CAD build for the part. Positions are in the model's coordinates, mm. Face numbers are marked on the shaded views. A direction names the side the tool comes from. Round coordinates to 2 decimals unless told otherwise and drop trailing zeros. Loops run counter-clockwise (first coordinate to the right, second up) from the corner with the lowest first, then second, coordinate; pieces in that order, holes last.
from build123d import *

# Parameters (mm, degrees)
SKETCH_1_W           = 50
SKETCH_1_H           = 50
EXTRUDE_1_DEPTH      = 220
EXTRUDE_2_DEPTH      = 50
SKETCH_4_W           = 37
SKETCH_4_H           = 37
CUT_EXTRUDE_2_DEPTH  = 12
CUT_EXTRUDE_3_REACH  = 235.922
SKETCH_5_R           = 8.5
SKETCH_8_R           = 0.75
CUT_EXTRUDE_4_DEPTH  = 6.5
CUT_EXTRUDE_START    = -6.5
SKETCH_7_R           = 0.75
CUT_EXTRUDE_5_DEPTH  = 6.5
CUT_EXTRUDE_6_DEPTH  = 5.5
CUT_EXTRUDE_7_DEPTH  = 5.5
CUT_EXTRUDE_8_DEPTH  = 50
FILLET_1_R           = 5
FILLET_2_R           = 5
FILLET_3_R           = 10
FILLET_4_R           = 10
SKETCH_13_W          = 47
SKETCH_13_H          = 47
CUT_EXTRUDE_9_DEPTH  = 50
SKETCH_2_W           = 43
SKETCH_2_H           = 43
CUT_EXTRUDE_10_DEPTH = 150
FILLET_5_R           = 5


with BuildPart() as part:
    # 草图1 → 凸台-拉伸1 (new body)
    with BuildSketch(Plane.XY):
        Rectangle(SKETCH_1_W, SKETCH_1_H)
    extrude(amount=EXTRUDE_1_DEPTH)

    # 草图3 → 凸台-拉伸2 (add)
    with BuildSketch(Plane(origin=(0, 25, 0), x_dir=(1, 0, 0), z_dir=(0, 1, 0))):
        Polygon((25, 0), (-25, 0), (26.961524227, 30), (76.961524227, 30), align=None)
    extrude(amount=-EXTRUDE_2_DEPTH)

    # 草图4 → 切除-拉伸2 (cut)
    with BuildSketch(Plane(origin=(6.25, 0, 10.825317547), x_dir=(0.8660254037844415, 0, -0.4999999999999951), z_dir=(0.4999999999999951, 0, 0.8660254037844415))):
        with Locations((41.650635095, 0)):
            Rectangle(SKETCH_4_W, SKETCH_4_H)
    extrude(amount=-CUT_EXTRUDE_2_DEPTH, mode=Mode.SUBTRACT)

    # 切除-拉伸3: up to this face of the body (flat: up to its plane)
    cut_extrude_3_end = Plane(part.part.faces().sort_by_distance((0.980762114, 0, -15))[0])
    # 草图5 → 切除-拉伸3 (cut, up to the picked face)
    with BuildSketch(Plane(origin=(0.25, 0, 0.433012702), x_dir=(0.8660254037844415, 0, -0.4999999999999951), z_dir=(0.4999999999999951, 0, 0.8660254037844415)), mode=Mode.PRIVATE) as cut_extrude_3_sk1:
        with Locations((45.150635095, 0)):
            Circle(SKETCH_5_R)
    cut_extrude_3_tool1 = split(extrude(cut_extrude_3_sk1.sketch, amount=-CUT_EXTRUDE_3_REACH, mode=Mode.PRIVATE), bisect_by=cut_extrude_3_end, keep=Keep.BOTH, mode=Mode.PRIVATE)
    add(cut_extrude_3_tool1.solids().sort_by(Axis((39.351597, 0, -22.142305), (-0.4999999999999951, 0, -0.8660254037844415)))[0], mode=Mode.SUBTRACT)

    # 草图8 → 切除-拉伸4 (cut)
    with BuildSketch(Plane.XZ.offset(-18.5)):
        with Locations((39.170508076, -15.455960044)):
            Circle(SKETCH_8_R)
    extrude(amount=-CUT_EXTRUDE_4_DEPTH, mode=Mode.SUBTRACT)

    # 草图7 → 切除-拉伸5 (cut)
    with BuildSketch(Plane(origin=(0, -18.5, 0), x_dir=(1, 0, 0), z_dir=(0, 1, 0)).offset(CUT_EXTRUDE_START)):
        with Locations((39.170508076, 15.455960044)):
            Circle(SKETCH_7_R)
    extrude(amount=CUT_EXTRUDE_5_DEPTH, mode=Mode.SUBTRACT)

    # 草图10 → 切除-拉伸6 (cut)
    with BuildSketch(Plane.XZ.offset(25)):
        Polygon((58.341978046, -19.25), (26.299038106, -0.75), (20.299038106, -11.142304845), (52.341978046, -29.642304845), align=None)
    extrude(amount=-CUT_EXTRUDE_6_DEPTH, mode=Mode.SUBTRACT)

    # 草图11 → 切除-拉伸7 (cut)
    with BuildSketch(Plane(origin=(0, 25, 0), x_dir=(1, 0, 0), z_dir=(0, 1, 0))):
        Polygon((26.299038106, 0.75), (58.341978046, 19.25), (52.341978046, 29.642304845), (20.299038106, 11.142304845), align=None)
    extrude(amount=-CUT_EXTRUDE_7_DEPTH, mode=Mode.SUBTRACT)

    # 草图12 → 切除-拉伸8 (cut)
    with BuildSketch(Plane.XZ.offset(25)):
        Polygon((64.404155872, -22.75), (60.218366421, -30), (76.961524227, -30), align=None)
    extrude(amount=-CUT_EXTRUDE_8_DEPTH, mode=Mode.SUBTRACT)

    # 圆角1
    fillet_1_edges = [part.edges().sort_by_distance(p)[0] for p in [
        (60.218366421, 0, -30),
    ]]
    fillet(fillet_1_edges, radius=FILLET_1_R)

    # 圆角2
    fillet_2_edges = [part.edges().sort_by_distance(p)[0] for p in [
        (26.961524227, -15.049152987, -30),
    ]]
    fillet(fillet_2_edges, radius=FILLET_2_R)

    # 圆角3
    fillet_3_edges = [part.edges().sort_by_distance(p)[0] for p in [
        (-25, 0, 0),
    ]]
    fillet(fillet_3_edges, radius=FILLET_3_R)

    # 圆角4
    # the kernel refuses this fillet: 10 mm, written as the material it adds along each edge
    with BuildSketch(Plane(origin=(25, 25, 0), x_dir=(0, 0, 1), z_dir=(0, -1, 0))) as fillet_4_piece_1_section:
        with BuildLine():
            CenterArc((FILLET_4_R * 0.57735026919, -FILLET_4_R), FILLET_4_R, 90, 60)
            Line((-FILLET_4_R * 0.288675134595, -FILLET_4_R * 0.5), (0, 0))
            Line((0, 0), (FILLET_4_R * 0.57735026919, 0))
        make_face()
    fillet_4_piece_1 = extrude(amount=50, mode=Mode.PRIVATE)
    fillet_4_piece_1 = split(fillet_4_piece_1, bisect_by=Plane(origin=(26.950281618, 22.25, 0.377986851), z_dir=(-0.8660254037844415, 0, 0.49999999999999517)), keep=Keep.TOP, mode=Mode.PRIVATE)
    add(fillet_4_piece_1)
    with BuildSketch(Plane(origin=(25, 39.43375673, 0), x_dir=(0, 0, 1), z_dir=(0, -1, 0))) as fillet_4_piece_2_section:
        with BuildLine():
            CenterArc((FILLET_4_R * 0.57735026919, -FILLET_4_R), FILLET_4_R, 90, 60)
            Line((-FILLET_4_R * 0.288675134595, -FILLET_4_R * 0.5), (0, 0))
            Line((0, 0), (FILLET_4_R * 0.57735026919, 0))
        make_face()
    fillet_4_piece_2 = extrude(amount=78.867513459, mode=Mode.PRIVATE)
    fillet_4_piece_2 = split(fillet_4_piece_2, bisect_by=Plane(origin=(27.357776316, 19.5, -1.0319296), z_dir=(0, -1, 0)), keep=Keep.TOP, mode=Mode.PRIVATE)
    fillet_4_piece_2 = split(fillet_4_piece_2, bisect_by=Plane(origin=(27.357776316, 18.5, -1.0319296), z_dir=(0, 1, 0)), keep=Keep.TOP, mode=Mode.PRIVATE)
    add(fillet_4_piece_2)
    with BuildSketch(Plane(origin=(25, 39.43375673, 0), x_dir=(0, 0, 1), z_dir=(0, -1, 0))) as fillet_4_piece_3_section:
        with BuildLine():
            CenterArc((FILLET_4_R * 0.57735026919, -FILLET_4_R), FILLET_4_R, 90, 60)
            Line((-FILLET_4_R * 0.288675134595, -FILLET_4_R * 0.5), (0, 0))
            Line((0, 0), (FILLET_4_R * 0.57735026919, 0))
        make_face()
    fillet_4_piece_3 = extrude(amount=78.867513459, mode=Mode.PRIVATE)
    fillet_4_piece_3 = split(fillet_4_piece_3, bisect_by=Plane(origin=(27.357776316, -19.5, -1.0319296), z_dir=(0, 1, 0)), keep=Keep.TOP, mode=Mode.PRIVATE)
    fillet_4_piece_3 = split(fillet_4_piece_3, bisect_by=Plane(origin=(27.357776316, -18.5, -1.0319296), z_dir=(0, -1, 0)), keep=Keep.TOP, mode=Mode.PRIVATE)
    add(fillet_4_piece_3)

    # 草图13 → 切除-拉伸9 (cut)
    with BuildSketch(Plane.XY.offset(220)):
        Rectangle(SKETCH_13_W, SKETCH_13_H)
    extrude(amount=-CUT_EXTRUDE_9_DEPTH, mode=Mode.SUBTRACT)

    # 草图2 → 切除-拉伸10 (cut)
    with BuildSketch(Plane.XY.offset(220)):
        Rectangle(SKETCH_2_W, SKETCH_2_H)
    extrude(amount=-CUT_EXTRUDE_10_DEPTH, mode=Mode.SUBTRACT)

    # 圆角5
    fillet_5_edges = [part.edges().sort_by_distance(p)[0] for p in [
        (26.961524227, 15.049152987, -30),
    ]]
    fillet(fillet_5_edges, radius=FILLET_5_R)


solid = part.part
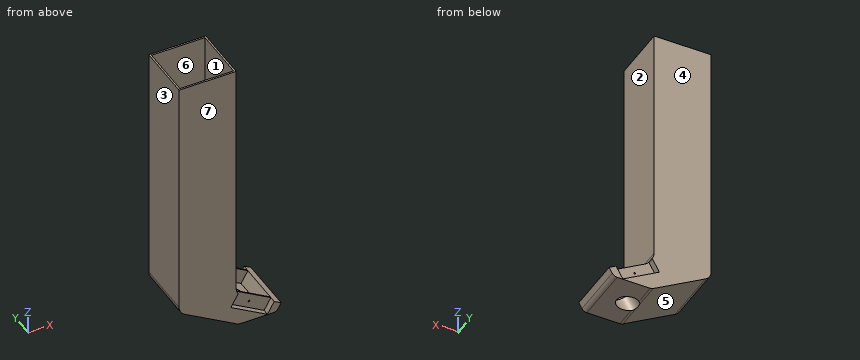
Item 1: Flat gauge pins, fed straight in: P1, Ø6, axis at x = 49, y = -18, coming from the +Z side; P2, Ø9, axis at x = 41, z = -11.5, coming from the +Y side; P3, Ø14, axis at x = 7.5, y = -3.5, coming from the +Z side; P4, Ø12, axis at x = 35.5, z = 119, coming from the +Y side. Where does each tip first touch, or does it go through?
Verdict:
P1: stops at z = -12.15
P2: stops at y = 19.5
P3: stops at z = 70
P4: passes through
Item 2: 3-axis set-ups, long thin cutter, end or side, ignore diameter. For the marked faces 1, 2 and 3: which of +Z, -Z, +X, -X, +Y, -Y reach the whole face in a straight line?
Verdict:
face 1: +Z
face 2: +Z, +X, +Y, -Y
face 3: +Z, -Z, -X, +Y, -Y
Item 3: Mould opens along Y. For the marked faces 4, 5, 6 and 7 say: released by +Y, released by -Y, zero draft, split by the parting line, or undercut.
Verdict:
face 4: released by +Y
face 5: zero draft
face 6: undercut
face 7: released by -Y
Item 4: Cut at B-B (x = -14). List the corners of the cut face in (y, z), plus the area to 3 significant figures.
Verdict:
outline: (-25, -6.35) - (25, -6.35) - (25, 220) - (23.5, 220) - (23.5, 170) - (21.5, 170) - (21.5, 70) - (-21.5, 70) - (-21.5, 170) - (-23.5, 170) - (-23.5, 220) - (-25, 220) - close
area: 4,670 mm2
Item 5: Wall check: L1, parallel to Y at x = 15, z = 178.5; L2, parallel to X at y = -5.5, z = 141. Give the ranges that are in metal, low to high.
Verdict:
L1: y = -25 to -23.5, 23.5 to 25
L2: x = -25 to -21.5, 21.5 to 25
Item 6: Cut at C-C (y = -13). List the corners of the cut face in (x, z).
Verdict:
outline: (-25, 5.77) arc R10 ccw to (-20, -2.89) - (25.8, -29.33) arc R5 ccw to (28.3, -30) - (57.33, -30) arc R5 ccw to (61.66, -27.5) - (64.4, -22.75) - (58.34, -19.25) - (52.34, -29.64) - (20.3, -11.14) - (26.78, 0.08) arc R10 cw to (25, 5.77) - (25, 220) - (23.5, 220) - (23.5, 170) - (21.5, 170) - (21.5, 70) - (-21.5, 70) - (-21.5, 170) - (-23.5, 170) - (-23.5, 220) - (-25, 220) - close
Item 7: Cut at D-D (z = 19). List the corners of the cut face in (x, y), plus the area to 3 significant figures.
Verdict:
outline: (-25, -25) - (25, -25) - (25, 25) - (-25, 25) - close
area: 2,500 mm2
Item 8: Cut at A-A (z = 106). List the corners of the cut face in (x, y), plus the area to 3 significant figures.
Verdict:
outline: (-25, -25) - (25, -25) - (25, 25) - (-25, 25) - close; hole (-21.5, -21.5) - (21.5, -21.5) - (21.5, 21.5) - (-21.5, 21.5) - close
area: 651 mm2
